Model file for the job. Use its own axes, mm. Face numbers are marked on the shaded views. Round coordinates to 2 decimals unless told otherwise and drop trailing zeros. Order: outer loops, then holes, each group sorted by start corner. A loop starts at its lowest first (then second) coordinate and runs counter-clockwise, first axis right, second up. Notation, with made-up numbers: (75.5, -29.5) - (115.5, -29.5) arc R19 cw to (115.5, -9.5) - close; hole circle Ø6 at (-26.5, 13.25). An arc over 180 degrees is marked (long way). Write item = value, one per line.
```python
from build123d import *

# Parameters (mm, degrees)
SKETCH1_W           = 50
SKETCH1_H           = 50
BOSS_EXTRUDE1_DEPTH = 8
SKETCH2_R           = 6
CUT_EXTRUDE2_DEPTH  = 4
SKETCH4_R           = 3.15
CUT_EXTRUDE3_DEPTH  = 4
FILLET1_R           = 4


with BuildPart() as part:
    # Sketch1 → Boss-Extrude1 (new body)
    with BuildSketch(Plane(origin=(0, 0, 0), x_dir=(1, 0, 0), z_dir=(0, 1, 0))):
        Rectangle(SKETCH1_W, SKETCH1_H)
    extrude(amount=BOSS_EXTRUDE1_DEPTH)

    # Sketch2 → Cut-Extrude2 (cut)
    with BuildSketch(Plane(origin=(0, 0, 0), x_dir=(1, 0, 0), z_dir=(0, 1, 0))):
        with Locations(Location((0, -12, 0), (0, 0, 270))):
            Circle(SKETCH2_R)
        with Locations(Location((0, 12, 0), (0, 0, 90))):
            Circle(SKETCH2_R)
    extrude(amount=CUT_EXTRUDE2_DEPTH, mode=Mode.SUBTRACT)

    # Sketch4 → Cut-Extrude3 (cut)
    with BuildSketch(Plane.XZ.offset(-4)):
        with Locations(Location((0, -12, 0), (0, 0, 270))):
            Circle(SKETCH4_R)
        with Locations(Location((0, 12, 0), (0, 0, 90))):
            Circle(SKETCH4_R)
    extrude(amount=-CUT_EXTRUDE3_DEPTH, mode=Mode.SUBTRACT)

    # Fillet1
    # the kernel refuses this fillet: 4 mm, written as the material it adds along each edge
    with BuildSketch(Plane(origin=(0, 4, 12), x_dir=(0, 0, 1), z_dir=(-1, 0, 0))) as fillet1_piece_1:
        with BuildLine():
            CenterArc((2, -3.831122551), FILLET1_R, 0, 73.291656284)
            Line((3.15, 0), (3.173, 0.076622451))
            ThreePointArc((3.173, 0.076622451), (4.575, 0.08), (6, 0.08))
            Line((6, 0.08), (6.08, 0))
            Line((6.08, 0), (6.08, -3.831122551))
            Line((6.08, -3.831122551), (6, -3.831122551))
        make_face()
    revolve(axis=Axis((0, 4, 12), (0, 1, 0)))
    with BuildSketch(Plane(origin=(0, 4, -12), x_dir=(0, 0, -1), z_dir=(1, 0, 0))) as fillet1_piece_2:
        with BuildLine():
            CenterArc((2, -3.831122551), FILLET1_R, 0, 73.291656284)
            Line((3.15, 0), (3.173, 0.076622451))
            ThreePointArc((3.173, 0.076622451), (4.575, 0.08), (6, 0.08))
            Line((6, 0.08), (6.08, 0))
            Line((6.08, 0), (6.08, -3.831122551))
            Line((6.08, -3.831122551), (6, -3.831122551))
        make_face()
    revolve(axis=Axis((0, 4, -12), (0, 1, 0)))


solid = part.part
```
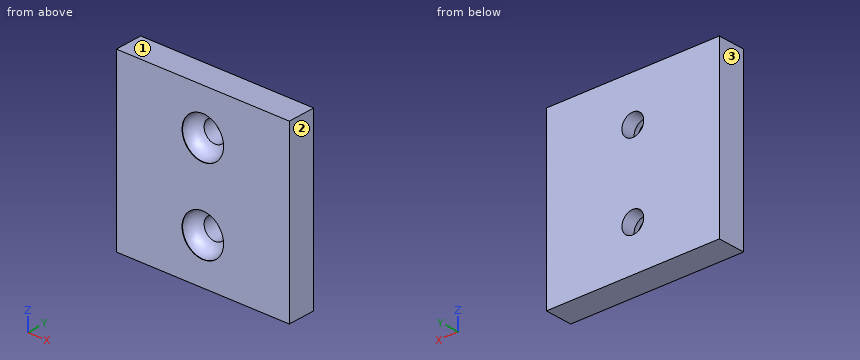
1) Mould opens along X. For the marked faces 1, 2 and 3 say: +X half, -X half, draft (parallel to the pull), parting line (faces both ways), or undercut.
Conclusion:
face_1 = draft
face_2 = +X half
face_3 = -X half
2) Flat gauge pins, fed straight in: pin 1 Ø11 at (x, z) = (0, 12) entering from +Y; pin 2 Ø7 at (x, z) = (0, 12) entering from -Y. Where does each tip first touch, or does it go through?
Conclusion:
pin_1 = 8
pin_2 = 3.88
3) Wall check: line 1 along Z through (x, y) = (2, 2); line 2 along X through (y, z) = (0.1, 12); line 3 along X through (y, z) = (4.5, -13). Give the ranges that are in metal, low to high.
Conclusion:
line_1 = -25 to -17.18, -6.82 to 6.82, 17.18 to 25
line_2 = -25 to -6, 6 to 25
line_3 = -25 to -2.99, 2.99 to 25
4) Cut at B-B (x = 0). Give the number of separate pieces and of enclosed holes in the cut face, and give its area (3 significant figures).
Conclusion:
separate_pieces = 3
enclosed_holes = 0
area = 265 mm^2
5) Cut at A-A (y = 6.25). Write the cut outline in (x, z), and give its area (3 significant figures).
Conclusion:
outline = (-25, -25) - (25, -25) - (25, 25) - (-25, 25) - close; hole circle Ø6.3 at (0, -12); hole circle Ø6.3 at (0, 12)
area = 2,440 mm^2
